from build123d import *

# Parameters (mm, degrees)
F0_W     = 100
F0_H     = 20
F1_DEPTH = 51
F2_W     = 20
F2_H     = 20
F3_DEPTH = 14
F5_D     = 3.3
F5_DEPTH = 7
F5_TIP   = 0.9914200214
F6_W     = 20
F6_H     = 20
F7_DEPTH = 25


with BuildPart() as f1:
    # F0 (on Top) → F1 (new body)
    with BuildSketch(Plane.XY):
        with Locations((50, 10)):
            Rectangle(F0_W, F0_H)
    extrude(amount=F1_DEPTH)

    # F2 (on face) → F3 (cut)
    with BuildSketch(Plane.XY.offset(51)):
        with Locations((10, 10)):
            Rectangle(F2_W, F2_H)
    extrude(amount=-F3_DEPTH, mode=Mode.SUBTRACT)

    # F5
    with Locations(Plane.XY.offset(37)):
        with Locations((5, 9), (15, 9)):
            Hole(F5_D / 2, depth=F5_DEPTH)
            with Locations((0, 0, -(F5_DEPTH + F5_TIP / 2))):  # 118° drill point
                Cone(0, F5_D / 2, F5_TIP, mode=Mode.SUBTRACT)

    # F6 (on face) → F7 (cut)
    with BuildSketch(Plane(origin=(0, 0, 0), x_dir=(1, 0, 0), z_dir=(0, 0, -1))):
        with Locations((10, -10)):
            Rectangle(F6_W, F6_H)
    extrude(amount=-F7_DEPTH, mode=Mode.SUBTRACT)


solid = f1.part
Input: part model. Units: mm. Frame: model coordinates. A direction names the side the tool comes from. Coordinates: 2 decimals unless noted, no trailing zeros. Loops run counter-clockwise (first coordinate to the right, second up) from the corner with the lowest first, then second, coordinate; pieces in that order, holes last.
(1) Pull-direction query (X, two-part tool) for faces 5 (the face through (20, 10, 12)), 6 (the face through (10, 10, 37)), 7 (the face through (5.15, 9.24, 29.18)); classes: released by +X, released by -X, zero draft, split by the parting line, or undercut.
(2) First-contact query: pin 1 Ø6 at (x, y) = (55, 15.5) entering from -Z; pin 2 Ø2 at (x, y) = (15, 9) entering from -Z; pin 3 Ø11 at (y, z) = (5.5, 45.5) entering from -X. Flat tips, straight axial feed; report the tip coordinate or a pass-through.
(3) Section A-A on y = 4.25. Return the cut outline in (x, z), then the cut area to 3 significant figures.
(4) Section B-B on z = 3.5. Return the cut outline in (x, y), then the cut area to 3 significant figures.
(5) Set-up query: faces 1 (the face through (10, 10, 25)), 2 (the face through (59, 10, 51)), 3 (the face through (20, 10, 44)), 4 (the face through (6.31, 8, 33.45)). Return all of +Z, -Z, +X, -X, +Y, -Y with unobstructed straight access to the full face (end or side cutting, diameter ignored); none if empty.
(6) Material intervals for probe 1 along X at (y, z) = (9, 32); probe 2 along Y at (x, z) = (5, 32.75); probe 3 along X at (y, z) = (5, 8), sorted ascending.
Data:
1. face 5: released by -X
1. face 6: zero draft
1. face 7: undercut
2. pin 1: stops at z = 0
2. pin 2: stops at z = 25
2. pin 3: stops at x = 20
3. outline: (0, 25) - (20, 25) - (20, 0) - (100, 0) - (100, 51) - (20, 51) - (20, 37) - (0, 37) - close
3. area: 4,320 mm2
4. outline: (20, 0) - (100, 0) - (100, 20) - (20, 20) - close
4. area: 1,600 mm2
5. face 1: -Z, -X, +Y, -Y
5. face 2: +Z, +X, -X, +Y, -Y
5. face 3: +Z, -X, +Y, -Y
5. face 4: +Z
6. probe 1: x = 0 to 3.35, 6.65 to 13.35, 16.65 to 100
6. probe 2: y = 0 to 7.35, 10.65 to 20
6. probe 3: x = 20 to 100
